from build123d import *

# Parameters (mm, degrees)
PAD019_DEPTH    = 10
POCKET027_DEPTH = 8
FILLET005_R     = 1
POCKET028_DEPTH = 27.344146
SKETCH089_W     = 2
SKETCH089_H     = 6.4
POCKET031_DEPTH = 3


with BuildPart() as part:
    # Sketch085 (on DatumPlane) → Pad019 (new body)
    with BuildSketch(Plane.XY.offset(18)):
        with BuildLine():
            Line((40, 105.4), (82, 105.4))
            ThreePointArc((88, 99.4), (86.242641, 103.642641), (82, 105.4))
            Line((88, 99.4), (88, 73.4))
            ThreePointArc((88, 73.4), (85.656854, 79.056854), (80, 81.4))
            Line((80, 81.4), (34, 81.4))
            Line((34, 81.4), (34, 99.4))
            ThreePointArc((40, 105.4), (35.757359, 103.642641), (34, 99.4))
        make_face()
    extrude(amount=-PAD019_DEPTH)

    # Sketch083 (on Face8 of Pad019) → Pocket027 (cut)
    with BuildSketch(Plane.XY.offset(16)):
        with BuildLine():
            Line((40, 103.4), (82, 103.4))
            ThreePointArc((86, 99.4), (84.828427, 102.228427), (82, 103.4))
            Line((86, 99.4), (86, 83.4))
            Line((86, 83.4), (36, 83.4))
            Line((36, 83.4), (36, 99.4))
            ThreePointArc((40, 103.4), (37.171573, 102.228427), (36, 99.4))
        make_face()
    extrude(amount=-POCKET027_DEPTH, mode=Mode.SUBTRACT)

    # Fillet005
    fillet005_edges = [part.edges().sort_by_distance(p)[0] for p in [
        (88, 73.4, 13),
    ]]
    fillet(fillet005_edges, radius=FILLET005_R)

    # Sketch086 (on DatumPlane) → Pocket028 (cut, through all)
    with BuildSketch(Plane(origin=(0, 105.4, 18), x_dir=(-1, 0, 0), z_dir=(0, 1, 0))):
        Polygon((-81.4, -3.8), (-40.6, -3.8), (-40.6, -5.2), (-39, -6.8), (-40.6, -8.4), (-40.6, -10), (-81.4, -10), (-81.4, -8.4), (-83, -6.8), (-81.4, -5.2), align=None)
    extrude(amount=-POCKET028_DEPTH, mode=Mode.SUBTRACT)

    # Sketch089 (on DatumPlane) → Pocket031 (cut)
    with BuildSketch(Plane(origin=(0, 0, 8), x_dir=(1, 0, 0), z_dir=(0, 0, -1))):
        with Locations((35, -89.6)):
            Rectangle(SKETCH089_W, SKETCH089_H)
        with Locations((87, -89.6)):
            Rectangle(SKETCH089_W, SKETCH089_H)
    extrude(amount=-POCKET031_DEPTH, mode=Mode.SUBTRACT)


solid = part.part
Could you check a few things on this model? Use its own coordinates, in mm. A direction names the side the tool comes from. Give positions to 0.01 mm unless a question says otherwise; leave off trailing zeros. Write each loop counter-clockwise with the first axis right and the second up, starting at its lowest first coordinate (ties: lowest second). Pieces come first, ordered by that corner, then holes. Notation, with made-up numbers: (6, 89.25) -> (16, 89.25) arc R5 cw to (16, 98.25) -> close; hole circle Ø2 at (39, 54). An arc over 180 degrees is marked (long way). Answer as a JSON object with one key per item and string values.
Q1. Suppose I cut it at C-C on x = 73. Write out the boundary of the cut face in (y, z).
Taken from the geometry:
{"outline": "(81.4, 14.2) -> (83.4, 14.2) -> (83.4, 16) -> (103.4, 16) -> (103.4, 14.2) -> (105.4, 14.2) -> (105.4, 18) -> (81.4, 18) -> close"}
Q2. Suppose I cut it at D-D on y = 82.5. Write out the boundary of the cut face in (x, z).
Taken from the geometry:
{"outline": "(34, 8) -> (40.6, 8) -> (40.6, 9.6) -> (39, 11.2) -> (40.6, 12.8) -> (40.6, 14.2) -> (81.4, 14.2) -> (81.4, 12.8) -> (83, 11.2) -> (81.4, 9.6) -> (81.4, 8) -> (88, 8) -> (88, 18) -> (34, 18) -> close"}
Q3. Which directions (+Z, -Z, +X, -X, +Y, -Y) give clear straight access to the entire face, cutting with the end or side of a thin tool? Please do faces 1 (the flat face through (82.2, 82.1, 12)), 2 (the flat face through (40.6, 104, 9)), 3 (the flat face through (87, 90, 11)), 4 (the flat face through (34, 90, 13)), 5 (the cylindrical face through (37.203, 102.259, 12.056)).
Taken from the geometry:
{"face 1": "+Y, -Y", "face 2": "-Z, +Y, -Y", "face 3": "-Z, +X, -X", "face 4": "+Z, -Z, -X, +Y, -Y", "face 5": "-Z"}
Q4. Please list where these lines run through material, in increasing order: L1, parallel to X at y = 99, z = 11.75; L2, parallel to Z at x = 49, y = 92; L3, parallel to Y at x = 50, z = 15.75.
Taken from the geometry:
{"L1": "x = 34 to 36, 86 to 88", "L2": "z = 16 to 18", "L3": "y = 81.4 to 83.4, 103.4 to 105.4"}
Q5. Will these pins go through, and if not, where does the flat tip stop? pin 1 Ø3 at (x, z) = (46, 13.5) entering from -Y; pin 2 Ø1.7 at (x, y) = (64.5, 82) entering from -Z; pin 3 Ø0.5 at (y, z) = (104, 8.5) entering from +X.
Taken from the geometry:
{"pin 1": "stops at y = 81.4", "pin 2": "stops at z = 14.2", "pin 3": "stops at x = 86.13"}
Q6. We'd pull the mould along X, two halves only. Please class faces 6 (the flat face through (61, 92, 18)), 7 (the flat face through (40.6, 82, 14)), 8 (the cylindrical face through (35.804, 103.689, 13.07)): released by +X, released by -X, zero draft, split by the parting line, or undercut.
Taken from the geometry:
{"face 6": "zero draft", "face 7": "undercut", "face 8": "released by -X"}
Q7. Suppose I cut it at B-B on y = 94.5. Write out the boundary of the cut face in (x, z), then the cut area to 3 significant figures.
Taken from the geometry:
{"outline": "(34, 8) -> (36, 8) -> (36, 16) -> (86, 16) -> (86, 8) -> (88, 8) -> (88, 18) -> (34, 18) -> close", "area": "140 mm²"}
Q8. Suppose I cut it at A-A on z = 9. Count the separate pieces of the cut face and the enclosed holes in it, then the cut area to 3 significant figures.
Taken from the geometry:
{"separate pieces": "4", "enclosed holes": "0", "area": "110 mm²"}
